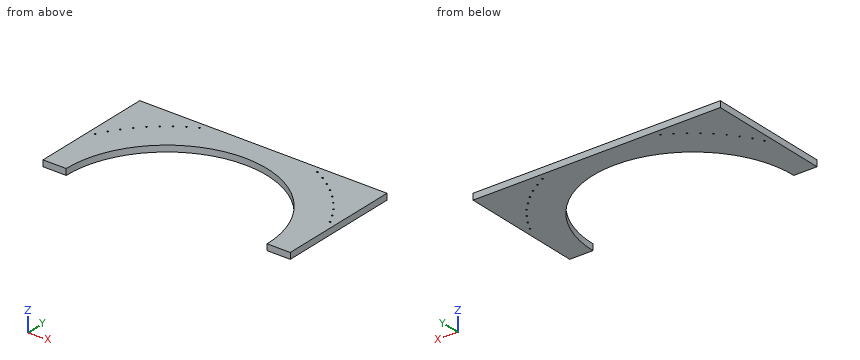
```python
from build123d import *

# Parameters (mm, degrees)
BOSS_EXTRU_1_DEPTH      = 2
ESQUISSE2_R             = 0.25
ENL_V_MAT_EXTRU_1_DEPTH = 2


with BuildPart() as part:
    # Esquisse1 → Boss.-Extru.1 (new body)
    with BuildSketch(Plane.XY):
        with BuildLine():
            Line((40, 0), (40, 40))
            Line((40, 40), (-40, 40))
            Line((-40, 40), (-40, 0))
            Line((-40, 0), (-32.5, 0))
            ThreePointArc((-32.5, 0), (0, 32.5), (32.5, 0))
            Line((32.5, 0), (40, 0))
        make_face()
    extrude(amount=BOSS_EXTRU_1_DEPTH)

    # Esquisse2 → Enlèv. mat.-Extru.1 (cut)
    with BuildSketch(Plane.XY.offset(2)):
        with Locations((-37.981453947, 19.069849399)):
            Circle(ESQUISSE2_R)
        with Locations((-36.335546301, 22.04491041)):
            Circle(ESQUISSE2_R)
        with Locations((-34.457091159, 24.878883995)):
            Circle(ESQUISSE2_R)
        with Locations((-32.358110634, 27.553632723)):
            Circle(ESQUISSE2_R)
        with Locations((-30.0520382, 30.0520382)):
            Circle(ESQUISSE2_R)
        with Locations((-27.553632723, 32.358110634)):
            Circle(ESQUISSE2_R)
        with Locations((-24.878883995, 34.457091159)):
            Circle(ESQUISSE2_R)
        with Locations((-22.04491041, 36.335546301)):
            Circle(ESQUISSE2_R)
        with Locations((-19.069849399, 37.981453947)):
            Circle(ESQUISSE2_R)
        with Locations(Location((19.069849399, 37.981453947, 0), (0, 0, 180))):
            Circle(ESQUISSE2_R)
        with Locations(Location((22.04491041, 36.335546301, 0), (0, 0, 180))):
            Circle(ESQUISSE2_R)
        with Locations(Location((24.878883995, 34.457091159, 0), (0, 0, 180))):
            Circle(ESQUISSE2_R)
        with Locations(Location((27.553632723, 32.358110634, 0), (0, 0, 180))):
            Circle(ESQUISSE2_R)
        with Locations(Location((30.0520382, 30.0520382, 0), (0, 0, 180))):
            Circle(ESQUISSE2_R)
        with Locations(Location((32.358110634, 27.553632723, 0), (0, 0, 180))):
            Circle(ESQUISSE2_R)
        with Locations(Location((34.457091159, 24.878883995, 0), (0, 0, 180))):
            Circle(ESQUISSE2_R)
        with Locations(Location((36.335546301, 22.04491041, 0), (0, 0, 180))):
            Circle(ESQUISSE2_R)
        with Locations(Location((37.981453947, 19.069849399, 0), (0, 0, 180))):
            Circle(ESQUISSE2_R)
    extrude(amount=-ENL_V_MAT_EXTRU_1_DEPTH, mode=Mode.SUBTRACT)


solid = part.part
```
Design review of the part built by this model. Coordinates are the model's own, in mm. Give positions to 0.01 mm unless a question says otherwise; leave off trailing zeros. Order: outer loops, then holes, each group sorted by start corner. A loop starts at its lowest first (then second) coordinate and runs counter-clockwise, first axis right, second up. Notation, with made-up numbers: (14.5, -31.75) -> (73.5, -31.75) arc R14 ccw to (73.5, -10.75) -> close; hole circle Ø9 at (37, -18). An arc over 180 degrees is marked (long way). Write item = value, one per line. Start each with the question number.
(1) We need section D-D on y = 21. Write out the cut boundary in (x, z).
(2) To check wall thickness, follow line 1 along X through (y, z) = (27.5, 0.65); line 2 along X through (y, z) = (27, 0.9); line 3 along X through (y, z) = (17.5, 0.9). State the ranges of each line that lie inside material, in increasing order.
(3) We need section A-A on y = 5. Write out the cut boundary in (x, z).
(4) We need section C-C on x = 0. Write out the cut boundary in (y, z).
(5) We need section B-B on z = 0.55. State how many separate pieces and enclosed holes the cut face has, plus the area to 3 significant figures.
Numbers:
q1.outline = (-40, 0) -> (-24.8, 0) -> (-24.8, 2) -> (-40, 2) -> close; (24.8, 0) -> (40, 0) -> (40, 2) -> (24.8, 2) -> close
q2.line_1 = -40 to -32.6, -32.11 to -17.32, 17.32 to 32.11, 32.6 to 40
q2.line_2 = -40 to -18.09, 18.09 to 40
q2.line_3 = -40 to -27.39, 27.39 to 40
q3.outline = (-40, 0) -> (-32.11, 0) -> (-32.11, 2) -> (-40, 2) -> close; (32.11, 0) -> (40, 0) -> (40, 2) -> (32.11, 2) -> close
q4.outline = (32.5, 0) -> (40, 0) -> (40, 2) -> (32.5, 2) -> close
q5.separate_pieces = 1
q5.enclosed_holes = 18
q5.area = 1,540 mm^2
